Print and shaded views of the part. All mm, measured from the part's lowest x, y and z. A direction names the side the tool comes from. Round coordinates to 2 decimals unless told otherwise and drop trailing zeros. Write each loop counter-clockwise with the first axis right and the second up, starting at its lowest first coordinate (ties: lowest second). Pieces come first, ordered by that corner, then holes. Notation, with made-up numbers: (-29.5, 84.25) -> (21.5, 84.25) arc R12 ccw to (21.5, 105.25) -> close; hole circle Ø6 at (-6.5, -21). An arc over 180 degrees is marked (long way). Return JSON: item names as keys, results as strings. Group by question number.
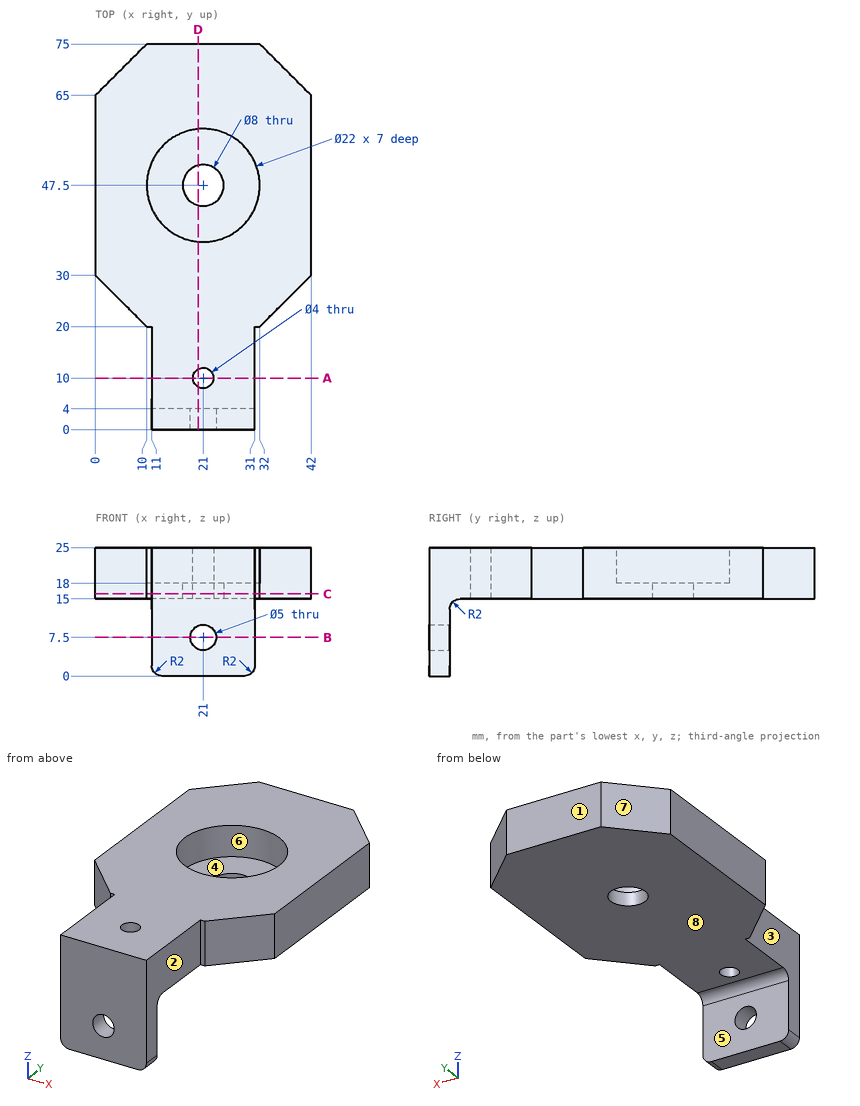
Item 1: Flat gauge pins, fed straight in: P1, Ø13, axis at x = 21, y = 47.5, coming from the +Z side; P2, Ø4, axis at x = 22, y = 56.5, coming from the +Z side; P3, Ø10, axis at y = 12.5, z = 13, coming from the +X side; P4, Ø6.5, axis at x = 22, z = 5, coming from the +Y side. Where does each tip first touch, or does it go through?
Item 2: Two-plate mould, pull along Y, no slides. Class the marked faces 6, 7 and 8: released by +Y, released by -Y, zero draft, split by the parting line, or undercut.
Item 3: Cut at C-C (z = 16). Write the cut outline in (x, y).
Item 4: Which spindle directions (+Z, -Z, +X, -X, +Y, -Y) get a long thin tool onto all of the face, cutting with end or side? Do the marked faces 1, 2, 3, 4 and 5. Say none if no direction does.
Item 5: Cut at B-B (z = 7.5). Write the cut outline in (x, y).
Item 6: Cut at A-A (y = 10). Write the cut outline in (x, z).
Item 7: Cut at D-D (x = 20). Write the cut outline in (y, z), then the cut area to 3 significant figures.
Item 8: Wall check: L1, parallel to Y at x = 21, z = 16.1; L2, parallel to Y at x = 21, z = 22.5; L3, parallel to X at y = 1.65, z = 7.5. Give the ranges that are in metal, low to high.
Checks:
{
 "1": {"P1": "stops at z = 18", "P2": "stops at z = 25", "P3": "stops at x = 31", "P4": "stops at y = 4"},
 "2": {"face 6": "undercut", "face 7": "released by +Y", "face 8": "zero draft"},
 "3": {"outline": "(0, 30) -> (10, 20) -> (11, 20) -> (11, 0) -> (31, 0) -> (31, 20) -> (32, 20) -> (42, 30) -> (42, 65) -> (32, 75) -> (10, 75) -> (0, 65) -> close; hole circle Ø8 at (21, 47.5); hole circle Ø4 at (21, 10)"},
 "4": {"face 1": "+Z, -Z, +X, -X, +Y", "face 2": "+Z, -Z, +X, -Y", "face 3": "+Z, -Z, -X, -Y", "face 4": "+Z", "face 5": "-Z, +X, -X, +Y"},
 "5": {"outline": "(11, 0) -> (18.5, 0) -> (18.5, 4) -> (11, 4) -> close; (23.5, 0) -> (31, 0) -> (31, 4) -> (23.5, 4) -> close"},
 "6": {"outline": "(11, 15) -> (19, 15) -> (19, 25) -> (11, 25) -> close; (23, 15) -> (31, 15) -> (31, 25) -> (23, 25) -> close"},
 "7": {"outline": "(0, 0) -> (4, 0) -> (4, 5.21) -> (0, 5.21) -> close; (0, 9.79) -> (4, 9.79) -> (4, 13) arc R2 cw to (6, 15) -> (8.27, 15) -> (8.27, 25) -> (0, 25) -> close; (11.73, 15) -> (43.63, 15) -> (43.63, 18) -> (36.55, 18) -> (36.55, 25) -> (11.73, 25) -> close; (51.37, 15) -> (75, 15) -> (75, 25) -> (58.45, 25) -> (58.45, 18) -> (51.37, 18) -> close", "area": "581 mm2"},
 "8": {"L1": "y = 0 to 8, 12 to 43.5, 51.5 to 75", "L2": "y = 0 to 8, 12 to 36.5, 58.5 to 75", "L3": "x = 11 to 18.5, 23.5 to 31"}
}
